Geometry: see drawing. Coordinates: mm, zero at the bounding-box minimum. Coordinates: 2 decimals unless noted, no trailing zeros. Write each loop counter-clockwise with the first axis right and the second up, starting at its lowest first coordinate (ties: lowest second). Pieces come first, ordered by that corner, then holes. Notation, with made-up numbers: (43.5, 17.25) - (50.5, 17.25) arc R22 ccw to (50.5, 35.25) - close; hole circle Ø6 at (15.5, -29.75). An arc over 180 degrees is marked (long way). Use CSV: the item, a comma, the result in double quotes.
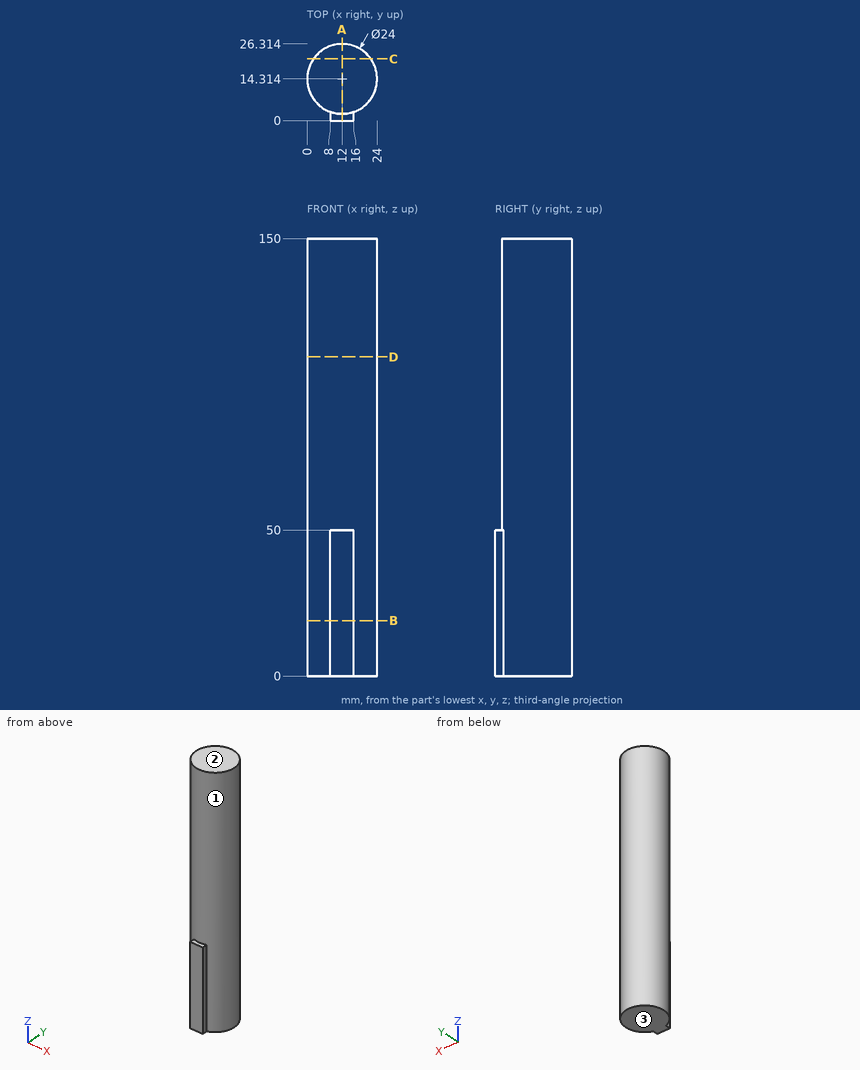
(1) Cut plane A-A on x = 12. Return loops of the section in (y, z), and give its area (3 significant figures).
Check values:
outline,"(0, 0) - (26.31, 0) - (26.31, 150) - (2.31, 150) - (2.31, 50) - (0, 50) - close"
area,"3,720 mm^2"
(2) Pin query (flat end, axial travel): pin 1 Ø3.5 at (y, z) = (1.5, 33.5) entering from +X (1 decimal); pin 2 Ø1.5 at (y, z) = (1.5, 30.5) entering from -X; pin 3 Ø4 at (y, z) = (9, 83) entering from -X. Return the tip coordinate at first contact, or that it passes through.
Check values:
pin 1,"x = 16.6"
pin 2,"x = 8"
pin 3,"x = 0.47"
(3) Ray query, probe 1 along X at (y, z) = (2.25, 33); probe 2 along Y at (x, z) = (13, 117) (1 decimal); probe 3 along Y at (x, z) = (8, 75.5). Return the intervals inside material, ascending. Write a range as from..to.
Check values:
probe 1,"8..16"
probe 2,"2.4..26.3"
probe 3,"3..25.63"
(4) Draft query along Z for the marked faces 1, 2 and 3. Return one class per face: pulls with the +Z half, pulls with the -Z half, needs draft (parallel to the pull), parting line crosses it, or undercut.
Check values:
face 1,"needs draft"
face 2,"pulls with the +Z half"
face 3,"pulls with the -Z half"
(5) Cut plane D-D on z = 109.5. Return loops of the section in (x, y), and give its area (3 significant figures).
Check values:
outline,"circle Ø24 at (12, 14.31)"
area,"452 mm^2"
(6) Cut plane C-C on y = 21.25. Return loops of the section in (x, z), and give its area (3 significant figures).
Check values:
outline,"(2.21, 0) - (21.79, 0) - (21.79, 150) - (2.21, 150) - close"
area,"2,940 mm^2"
(7) Cut plane B-B on z = 19. Return loops of the section in (x, y).
Check values:
outline,"(8, 0) - (16, 0) - (16, 3) arc R12 ccw (long way) to (8, 3) - close"
